Study the drawing (mm; zero at the part's minimum x, y, z) and answer. A direction names the side the tool comes from. Give positions to 0.01 mm unless a question says otherwise; leave off trailing zeros. Write each loop counter-clockwise with the first axis right and the second up, starting at its lowest first coordinate (ties: lowest second). Pieces come first, ordered by that corner, then holes.
1) Find section A-A (y = 25). Determine the outline of the cut face in (x, z).
2) A tool of negligible diameter and unlimited length cuts with its end or side. For the marked faces 5, 6 and 7, from which of +Z, -Z, +X, -X, +Y, -Y can it reach the whole face along a straight path? Write none if from no direction.
3) Find section B-B (x = 5). Determine the outline of the cut face in (y, z).
4) Straight lines are drawn through the part: probe 1 along Y at (x, z) = (5, 1.75); probe 2 along X at (y, z) = (19.25, 24.5); probe 3 along X at (y, z) = (26.5, 46.5). For each, find the intervals that lie inside material, in ascending order.
5) Determine the mould class of the marked faces 1, 2, 3 and 4 for opening direction X: pulls with the +X half, pulls with the -X half, needs draft (parallel to the pull), parting line crosses it, or undercut.
6) Find section D-D (z = 12.5). Determine the outline of the cut face in (x, y), plus the area to 3 significant figures.
7) Given pin 1 Ø6 at (x, y) = (4, 21) entering from +Z; pin 2 Ø12 at (x, z) = (30.5, 34.5) entering from -Y; pin 3 Ø2.5 at (x, y) = (65, 5) entering from +Z; pin 4 Ø1.5 at (y, z) = (15, 41.5) entering from -X, each flat-ended and moving along its own axis, determine where each tip first touches the part or whether it passes through.
8) Find section C-C (y = 5). Determine the outline of the cut face in (x, z).
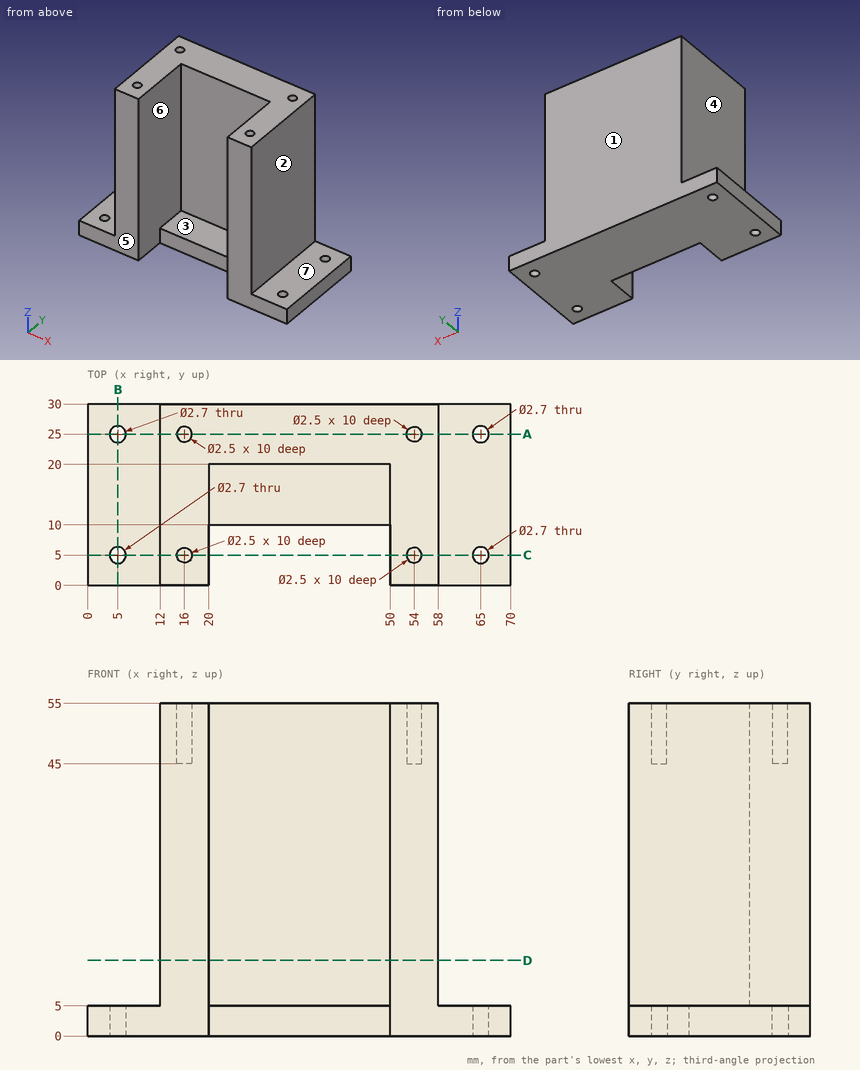
Results:
1. outline: (0, 0) - (3.65, 0) - (3.65, 5) - (0, 5) - close; (6.35, 0) - (63.65, 0) - (63.65, 5) - (58, 5) - (58, 55) - (55.25, 55) - (55.25, 45) - (52.75, 45) - (52.75, 55) - (17.25, 55) - (17.25, 45) - (14.75, 45) - (14.75, 55) - (12, 55) - (12, 5) - (6.35, 5) - close; (66.35, 0) - (70, 0) - (70, 5) - (66.35, 5) - close
2. face 5: +Z, -Z, +X, -X, -Y
2. face 6: +Z, -Y
2. face 7: +Z, +X, +Y, -Y
3. outline: (0, 0) - (3.65, 0) - (3.65, 5) - (0, 5) - close; (6.35, 0) - (23.65, 0) - (23.65, 5) - (6.35, 5) - close; (26.35, 0) - (30, 0) - (30, 5) - (26.35, 5) - close
4. probe 1: y = 0 to 3.65, 6.35 to 23.65, 26.35 to 30
4. probe 2: x = 12 to 20, 50 to 58
4. probe 3: x = 12 to 58
5. face 1: needs draft
5. face 2: pulls with the +X half
5. face 3: undercut
5. face 4: pulls with the -X half
6. outline: (12, 0) - (20, 0) - (20, 20) - (50, 20) - (50, 0) - (58, 0) - (58, 30) - (12, 30) - close
6. area: 780 mm2
7. pin 1: stops at z = 5
7. pin 2: stops at y = 20
7. pin 3: passes through
7. pin 4: stops at x = 12
8. outline: (0, 0) - (3.65, 0) - (3.65, 5) - (0, 5) - close; (6.35, 0) - (20, 0) - (20, 55) - (17.25, 55) - (17.25, 45) - (14.75, 45) - (14.75, 55) - (12, 55) - (12, 5) - (6.35, 5) - close; (50, 0) - (63.65, 0) - (63.65, 5) - (58, 5) - (58, 55) - (55.25, 55) - (55.25, 45) - (52.75, 45) - (52.75, 55) - (50, 55) - close; (66.35, 0) - (70, 0) - (70, 5) - (66.35, 5) - close
